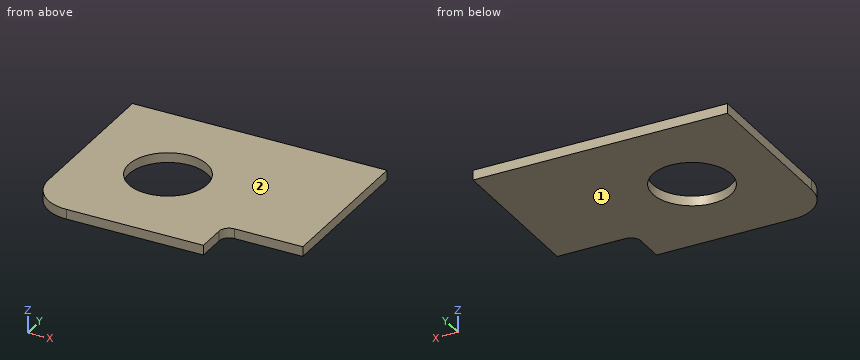
```python
from build123d import *

# Parameters (mm, degrees)
SKIZZE1_R                       = 20
AUFSATZ_LINEAR_AUSTRAGEN1_DEPTH = 5


with BuildPart() as part:
    # Skizze1 → Aufsatz-Linear austragen1 (new body)
    with BuildSketch(Plane.XY):
        with BuildLine():
            Line((20, 0), (90, 0))
            Line((90, 0), (90, 15))
            ThreePointArc((90, 15), (91.464466094, 18.535533906), (95, 20))
            Line((95, 20), (130, 20))
            Line((130, 20), (130, 100))
            Line((130, 100), (0, 100))
            Line((0, 100), (0, 20))
            ThreePointArc((0, 20), (5.857864376, 5.857864376), (20, 0))
        make_face()
        with Locations((45, 50)):
            Circle(SKIZZE1_R, mode=Mode.SUBTRACT)
    extrude(amount=AUFSATZ_LINEAR_AUSTRAGEN1_DEPTH)


solid = part.part
```
Geometry check sheet. Reference: the model listing, model coordinates, mm. Face numbers are marked on the shaded views. Coordinates: 2 decimals unless noted, no trailing zeros. Order: outer loops, then holes, each group sorted by start corner. A loop starts at its lowest first (then second) coordinate and runs counter-clockwise, first axis right, second up. Notation, with made-up numbers: (19, 34.5) - (57, 34.5) arc R21 ccw to (57, 70.5) - close; hole circle Ø7 at (52, 59). An arc over 180 degrees is marked (long way). Answer as a JSON object with one key per item and string values. Group by question number.
Item 1: Sectioned sample at D-D, the plane x = 121.5. Record the cut outline in (y, z), and give its area (3 significant figures).
Item 2: Depth check by flat-ended pin: pin 1 Ø2.5 at (y, z) = (7, 3) entering from +X. Enter the tip coordinate at first touch or a pass-through.
Item 3: Sectioned sample at A-A, the plane y = 50. Record the cut outline in (x, z), and give its area (3 significant figures).
Item 4: Draft check along Z on the marked faces 1 and 2. Enter one of: +Z half, -Z half, draft (parallel to the pull), parting line (faces both ways), or undercut.
Item 5: Scan lines: probe 1 along Y at (x, z) = (45, 2.8); probe 2 along Y at (x, z) = (19.5, 3.7); probe 3 along X at (y, z) = (68.5, 3.4). Record each from-to range of solid material in increasing order.
Item 6: Sectioned sample at C-C, the plane x = 45. Record the cut outline in (y, z), and give its area (3 significant figures).
Item 7: Sectioned sample at B-B, the plane z = 1.2. Record the cut outline in (x, y).
Resolved:
{
 "1": {"outline": "(20, 0) - (100, 0) - (100, 5) - (20, 5) - close", "area": "400 mm^2"},
 "2": {"pin 1": "x = 90"},
 "3": {"outline": "(0, 0) - (25, 0) - (25, 5) - (0, 5) - close; (65, 0) - (130, 0) - (130, 5) - (65, 5) - close", "area": "450 mm^2"},
 "4": {"face 1": "-Z half", "face 2": "+Z half"},
 "5": {"probe 1": "0 to 30, 70 to 100", "probe 2": "0.01 to 100", "probe 3": "0 to 37.4, 52.6 to 130"},
 "6": {"outline": "(0, 0) - (30, 0) - (30, 5) - (0, 5) - close; (70, 0) - (100, 0) - (100, 5) - (70, 5) - close", "area": "300 mm^2"},
 "7": {"outline": "(0, 20) arc R20 ccw to (20, 0) - (90, 0) - (90, 15) arc R5 cw to (95, 20) - (130, 20) - (130, 100) - (0, 100) - close; hole circle Ø40 at (45, 50)"}
}
